```python
from build123d import *

# Parameters (mm, degrees)
F2_SIZE = 5.08
F3_R    = 5.08


with BuildPart() as f1:
    # F0 (on Front) → F1 (revolve)
    with BuildSketch(Plane.XZ):
        Polygon((-30.128215, 18.680663), (-49.528385, 12.636178), (-50.8, 0), (0, 0), (-9.342636, 8.602624), (-9.342636, 59.402624), align=None)
    revolve(axis=Axis((-25.4, 0, 0), (-1, 0, 0)))

    # F2
    f2_edges = [f1.edges().sort_by_distance(p)[0] for p in [
        (-9.342636, 0, -8.602624),
        (-4.671318, 0, 4.301312),
    ]]
    chamfer(f2_edges, length=F2_SIZE)

    # F3
    f3_edges = [f1.edges().sort_by_distance(p)[0] for p in [
        (-49.528385, 0, -12.636178),
        (-50.164193, 0, 6.318089),
    ]]
    fillet(f3_edges, radius=F3_R)


solid = f1.part
```
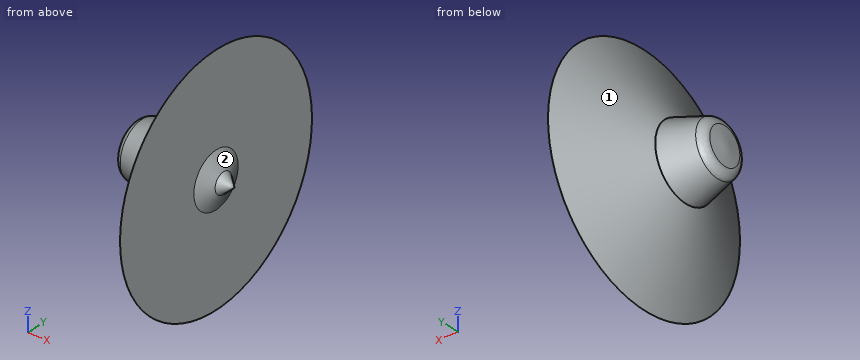
Part model, mm, in its own coordinate system. Face numbers are marked on the shaded views. Give positions to 0.01 mm unless a question says otherwise; leave off trailing zeros. Loops run counter-clockwise (first coordinate to the right, second up) from the corner with the lowest first, then second, coordinate; pieces in that order, holes last. Notation, with made-up numbers: M 68.5,-29 L 125.5,-29 A8 ccw 125.5,-25 Z; hole C 7,15.25 d7. An arc over 180 degrees is marked long. Return JSON: item names as keys, results as strings.
1) Saw through at A-A, the plane x = -32. List the corners of the cut face in (y, z), then the cut area to 3 significant figures.
Calculated:
{"outline": "C 0,0 d36.19", "area": "1,030 mm2"}
2) Pull direction X, two halves, no side cores. Call the marked faces 1 and 2: released by +X, released by -X, zero draft, split by the parting line, or undercut.
Calculated:
{"face 1": "released by -X", "face 2": "released by +X"}
3) Saw through at B-B, the plane x = -22. List the corners of the cut face in (y, z).
Calculated:
{"outline": "C 0,0 d69.21"}
4) Drill centre lines: line 1 (Y direction, x = -40, z = 10); line 2 (X direction, y = -35, z = -42.5); line 3 (X direction, y = 9, z = 7). Where is each one in solid material? Low to high.
Calculated:
{"line 1": "y = -11.98 to 11.98", "line 2": "x = -11.56 to -9.34", "line 3": "x = -49.16 to -8.34"}
5) Flat gauge pins, fed straight in: pin 1 Ø8 at (y, z) = (-44.5, 37) entering from -X; pin 2 Ø10 at (y, z) = (-33, 33) entering from -X; pin 3 Ø12 at (y, z) = (28.5, 16) entering from -X. Where does each tip first touch, or does it go through?
Calculated:
{"pin 1": "stops at x = -12.17", "pin 2": "stops at x = -18.39", "pin 3": "stops at x = -26.04"}
